from build123d import *

# Parameters (mm, degrees)
BOSS_EXTRUDE1_DEPTH = 3
SKETCH2_W           = 9
SKETCH2_H           = 11
CUT_EXTRUDE1_DEPTH  = 3
SKETCH3_W           = 14
SKETCH3_H           = 9
CUT_EXTRUDE2_DEPTH  = 3


with BuildPart() as part:
    # Sketch1 → Boss-Extrude1 (new body)
    with BuildSketch(Plane.XY):
        Polygon((25, 28), (25, 25), (35, 25), (35, 28), (45, 28), (45, 25), (45, 15), (48, 15), (48, 5), (45, 5), (45, -5), (48, -5), (48, -15), (45, -15), (45, -25), (45, -28), (35, -28), (35, -25), (25, -25), (25, -28), (15, -28), (15, -25), (5, -25), (5, -28), (-5, -28), (-5, -25), (-15, -25), (-15, -28), (-25, -28), (-25, -25), (-35, -25), (-35, -28), (-45, -28), (-45, -25), (-45, -15), (-48, -15), (-48, -5), (-45, -5), (-45, 5), (-48, 5), (-48, 15), (-45, 15), (-45, 25), (-45, 28), (-35, 28), (-35, 25), (-25, 25), (-25, 28), (-15, 28), (-15, 25), (-5, 25), (-5, 28), (5, 28), (5, 25), (15, 25), (15, 28), align=None)
    extrude(amount=BOSS_EXTRUDE1_DEPTH)

    # Sketch2 → Cut-Extrude1 (cut)
    with BuildSketch(Plane.XY.offset(3)):
        with Locations((19.5, -7.5)):
            Rectangle(SKETCH2_W, SKETCH2_H)
    extrude(amount=-CUT_EXTRUDE1_DEPTH, mode=Mode.SUBTRACT)

    # Sketch3 → Cut-Extrude2 (cut)
    with BuildSketch(Plane.XY.offset(3)):
        Rectangle(SKETCH3_W, SKETCH3_H)
    extrude(amount=-CUT_EXTRUDE2_DEPTH, mode=Mode.SUBTRACT)


solid = part.part
For this review, take the finished solid that the model builds, in its own axes (mm). A direction names the side the tool comes from. Coordinates: 2 decimals unless noted, no trailing zeros. Order: outer loops, then holes, each group sorted by start corner. A loop starts at its lowest first (then second) coordinate and runs counter-clockwise, first axis right, second up. Notation, with made-up numbers: (58, 55) -> (65, 55) arc R24 ccw to (65, 84) -> close; hole circle Ø9 at (-14.75, 86). An arc over 180 degrees is marked (long way). Return JSON: item names as keys, results as strings.
1. Machinability: for faces 1 (the flat face through (-7, 0, 2)), 2 (the flat face through (-15, 27, 1)), 3 (the flat face through (47, -15, 1)), which of the approach directions +Z, -Z, +X, -X, +Y, -Y give a long, thin tool a straight path to every point of the face, cutting with its end or side? Answer none if there is none.
Answer block:
{"face 1": "+Z, -Z", "face 2": "+Z, -Z, +Y", "face 3": "+Z, -Z, +X, -Y"}
2. The part is to be moulded in two halves that separate along X. For faces 4 (the flat face through (-5, 26, 1)), 5 (the flat face through (46, 15, 1)), 6 (the flat face through (48, -10, 1)), say which applies: +X half, -X half, draft (parallel to the pull), parting line (faces both ways), or undercut.
Answer block:
{"face 4": "undercut", "face 5": "draft", "face 6": "+X half"}
3. We need section D-D on y = -24. Write out the cut boundary in (x, z), and give its area (3 significant figures).
Answer block:
{"outline": "(-45, 0) -> (45, 0) -> (45, 3) -> (-45, 3) -> close", "area": "270 mm²"}
4. We need section A-A on x = 23. Write out the cut boundary in (y, z), and give its area (3 significant figures).
Answer block:
{"outline": "(-28, 0) -> (-13, 0) -> (-13, 3) -> (-28, 3) -> close; (-2, 0) -> (28, 0) -> (28, 3) -> (-2, 3) -> close", "area": "135 mm²"}
5. For pin 1 Ø1.5 at (x, z) = (-46, 1) entering from -Y; pin 2 Ø0.9 at (y, z) = (-26, 2) entering from +X; pin 3 Ø1.5 at (y, z) = (26, 1.5) entering from -X; pin 4 Ø4 at (x, y) = (-5.5, -4.5) entering from -Z, all flat-tipped, find the tip position at first contact; note any pin that passes through.
Answer block:
{"pin 1": "y = -15", "pin 2": "x = 45", "pin 3": "x = -45", "pin 4": "z = 0"}
6. For line 1 (X direction, y = 25.5, z = 1.7); line 2 (X direction, y = -8, z = 2.2); line 3 (Y direction, x = -14, z = 0.9), list the stretches that pass through material, from the lowest coordinate up. Write a range as from..to.
Answer block:
{"line 1": "-45..-35, -25..-15, -5..5, 15..25, 35..45", "line 2": "-48..15, 24..48", "line 3": "-25..25"}
7. We need section C-C on z = 0.85. State how many separate pieces and enclosed holes the cut face has, and give its area (4 significant figures).
Answer block:
{"separate pieces": "1", "enclosed holes": "2", "area": "4,695 mm²"}
8. We need section B-B on y = -6.5. Write out the cut boundary in (x, z).
Answer block:
{"outline": "(-48, 0) -> (15, 0) -> (15, 3) -> (-48, 3) -> close; (24, 0) -> (48, 0) -> (48, 3) -> (24, 3) -> close"}
